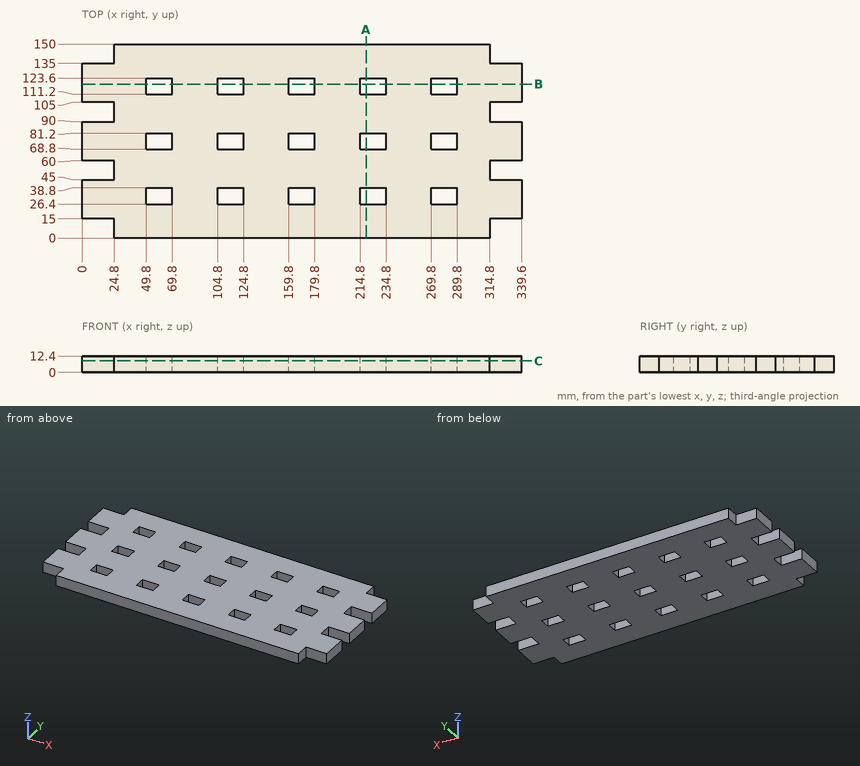
Design review of the part shown in the three views and the two pictorial views. Dimensions are in mm from the part's minimum x, y and z. Round coordinates to 2 decimals unless told otherwise and drop trailing zeros. Order: outer loops, then holes, each group sorted by start corner. A loop starts at its lowest first (then second) coordinate and runs counter-clockwise, first axis right, second up.
Q1. We need section C-C, the plane z = 8.75. State how many separate pieces and enclosed holes the cut face has, plus the area to 3 significant figures.
Findings below:
separate pieces: 1
enclosed holes: 15
area: 44,200 mm2
Q2. We need section B-B, the plane y = 119. Give the boundary of the cut face in (x, z), plus the area to 3 significant figures.
Findings below:
outline: (0, 0) - (49.8, 0) - (49.8, 12.4) - (0, 12.4) - close; (69.8, 0) - (104.8, 0) - (104.8, 12.4) - (69.8, 12.4) - close; (124.8, 0) - (159.8, 0) - (159.8, 12.4) - (124.8, 12.4) - close; (179.8, 0) - (214.8, 0) - (214.8, 12.4) - (179.8, 12.4) - close; (234.8, 0) - (269.8, 0) - (269.8, 12.4) - (234.8, 12.4) - close; (289.8, 0) - (339.6, 0) - (339.6, 12.4) - (289.8, 12.4) - close
area: 2,970 mm2
Q3. We need section A-A, the plane x = 219.5. Give the boundary of the cut face in (y, z).
Findings below:
outline: (0, 0) - (26.4, 0) - (26.4, 12.4) - (0, 12.4) - close; (38.8, 0) - (68.8, 0) - (68.8, 12.4) - (38.8, 12.4) - close; (81.2, 0) - (111.2, 0) - (111.2, 12.4) - (81.2, 12.4) - close; (123.6, 0) - (150, 0) - (150, 12.4) - (123.6, 12.4) - close
Q4. Wall thickness on line 1 (X direction, y = 29, z = 8.5); line 2 (Y direction, x = 122.5, z = 10.5); line 3 (X direction, y = 47, z = 5.5): over which ranges is each line inside the solid? List them lowest first.
Findings below:
line 1: x = 0 to 49.8, 69.8 to 104.8, 124.8 to 159.8, 179.8 to 214.8, 234.8 to 269.8, 289.8 to 339.6
line 2: y = 0 to 26.4, 38.8 to 68.8, 81.2 to 111.2, 123.6 to 150
line 3: x = 24.8 to 314.8
Q5. Insertion check: P1, Ø6, axis at x = 169, z = 8, coming from the -Y side; P2, Ø6, axis at x = 15.5, z = 6.5, coming from the -Y side. Each pin has a flat end and moves straight along its axis. Give the tip position at first contact, or say it passes through.
Findings below:
P1: stops at y = 0
P2: stops at y = 15
